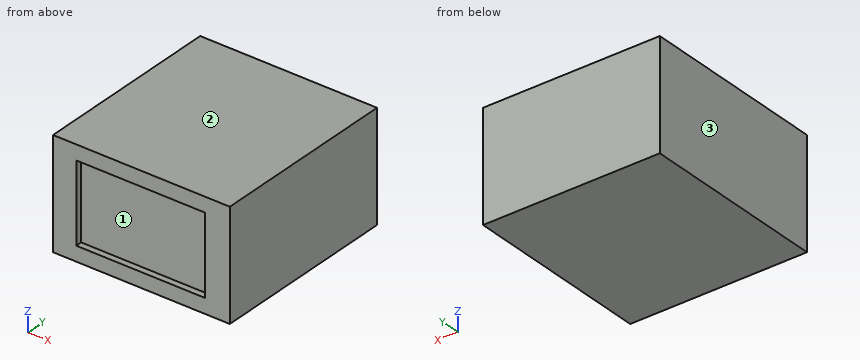
from build123d import *

# Parameters (mm, degrees)
SKETCH_W     = 140
SKETCH_H     = 150
PAD_DEPTH    = 86
SKETCH001_W  = 102.094734
SKETCH001_H  = 62.564154
POCKET_DEPTH = 5


with BuildPart() as part:
    # Sketch → Pad (new body)
    with BuildSketch(Plane.XY):
        with Locations((70, -75)):
            Rectangle(SKETCH_W, SKETCH_H)
    extrude(amount=PAD_DEPTH)

    # Sketch001 (on Face3 of Pad) → Pocket (cut)
    with BuildSketch(Plane.XZ.offset(150)):
        with Locations((69.496113, 43.012418)):
            Rectangle(SKETCH001_W, SKETCH001_H)
    extrude(amount=-POCKET_DEPTH, mode=Mode.SUBTRACT)


solid = part.part
For this review, take the finished solid that the model builds, in its own axes (mm). Face numbers are marked on the shaded views. Coordinates: 2 decimals unless noted, no trailing zeros. Order: outer loops, then holes, each group sorted by start corner. A loop starts at its lowest first (then second) coordinate and runs counter-clockwise, first axis right, second up. Notation, with made-up numbers: (-9.75, 87.5) -> (48.25, 87.5) arc R10 ccw to (48.25, 95.5) -> close; hole circle Ø4 at (12, 38). An arc over 180 degrees is marked (long way). Return JSON: item names as keys, results as strings.
1. We need section B-B on z = 23. Write out the cut boundary in (x, y).
Answer block:
{"outline": "(0, -150) -> (18.45, -150) -> (18.45, -145) -> (120.54, -145) -> (120.54, -150) -> (140, -150) -> (140, 0) -> (0, 0) -> close"}
2. We need section A-A on x = 116.5. Write out the cut boundary in (y, z), and give its area (3 significant figures).
Answer block:
{"outline": "(-150, 0) -> (0, 0) -> (0, 86) -> (-150, 86) -> (-150, 74.29) -> (-145, 74.29) -> (-145, 11.73) -> (-150, 11.73) -> close", "area": "12,600 mm²"}
3. The part is to be moulded in two halves that separate along X. For the marked faces 1, 2 and 3, say which applies: +X half, -X half, draft (parallel to the pull), parting line (faces both ways), or undercut.
Answer block:
{"face 1": "undercut", "face 2": "draft", "face 3": "-X half"}
4. For line 1 (Y direction, x = 20, z = 49.5), list the stretches that pass through material, from the lowest coordinate up. Write a range as from..to.
Answer block:
{"line 1": "-145..0"}
